The listing builds one solid part. Answer for the finished solid, in the listing's coordinates (mm). Give positions to 0.01 mm unless a question says otherwise; leave off trailing zeros. Write each loop counter-clockwise with the first axis right and the second up, starting at its lowest first coordinate (ties: lowest second). Pieces come first, ordered by that corner, then holes.
```python
from build123d import *

# Parameters (mm, degrees)
SKETCH1_W           = 609.6
SKETCH1_H           = 609.6
BOSS_EXTRUDE1_DEPTH = 6.35
SKETCH2_R           = 6.35
CUT_EXTRUDE1_DEPTH  = 6.35
SKETCH3_W           = 304.8
SKETCH3_H           = 304.8
CUT_EXTRUDE2_DEPTH  = 432.099063441
SKETCH4_R           = 3.175
CUT_EXTRUDE3_DEPTH  = 432.099063441


with BuildPart() as part:
    # Sketch1 → Boss-Extrude1 (new body)
    with BuildSketch(Plane.XY):
        Rectangle(SKETCH1_W, SKETCH1_H)
    extrude(amount=BOSS_EXTRUDE1_DEPTH)

    # Sketch2 → Cut-Extrude1 (cut)
    with BuildSketch(Plane.XY.offset(6.35)):
        with Locations((254, -254)):
            Circle(SKETCH2_R)
    extrude(amount=-CUT_EXTRUDE1_DEPTH, mode=Mode.SUBTRACT)

    # Sketch3 → Cut-Extrude2 (cut, through all)
    with BuildSketch(Plane.XY.offset(6.35)):
        Rectangle(SKETCH3_W, SKETCH3_H)
    extrude(amount=-CUT_EXTRUDE2_DEPTH, mode=Mode.SUBTRACT)

    # Sketch4 → Cut-Extrude3 (cut, through all)
    with BuildSketch(Plane.XY.offset(6.35)):
        with Locations((-266.7, -266.7)):
            Circle(SKETCH4_R)
    extrude(amount=-CUT_EXTRUDE3_DEPTH, mode=Mode.SUBTRACT)


solid = part.part
```
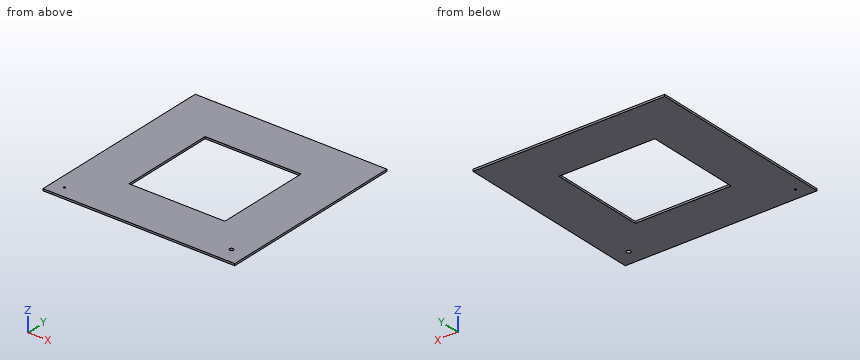
Item 1: A cutting plane is placed at A-A, the plane x = -145.5. Give the vertices of the cut face in (y, z), plus the area to 3 significant figures.
Conclusion:
outline: (-304.8, 0) - (-152.4, 0) - (-152.4, 6.35) - (-304.8, 6.35) - close; (152.4, 0) - (304.8, 0) - (304.8, 6.35) - (152.4, 6.35) - close
area: 1,940 mm2
Item 2: A cutting plane is placed at B-B, the plane z = 3.5. Give the vertices of the cut face in (x, y) (3 decimals).
Conclusion:
outline: (-304.8, -304.8) - (304.8, -304.8) - (304.8, 304.8) - (-304.8, 304.8) - close; hole circle Ø6.35 at (-266.7, -266.7); hole (-152.4, -152.4) - (152.4, -152.4) - (152.4, 152.4) - (-152.4, 152.4) - close; hole circle Ø12.7 at (254, -254)
Item 3: Consider probe 1 along Y at (x, z) = (254, 4); probe 2 along X at (y, z) = (141.5, 5.5); probe 3 along X at (y, z) = (-266.7, 4.5) (3 decimals). Determine where each line is inside the solid, lowest interval first.
Conclusion:
probe 1: y = -304.8 to -260.35, -247.65 to 304.8
probe 2: x = -304.8 to -152.4, 152.4 to 304.8
probe 3: x = -304.8 to -269.875, -263.525 to 304.8
